Geometry check sheet. Reference: the model listing, model coordinates, mm. Face numbers are marked on the shaded views. A direction names the side the tool comes from. Round coordinates to 2 decimals unless told otherwise and drop trailing zeros. Loops run counter-clockwise (first coordinate to the right, second up) from the corner with the lowest first, then second, coordinate; pieces in that order, holes last.
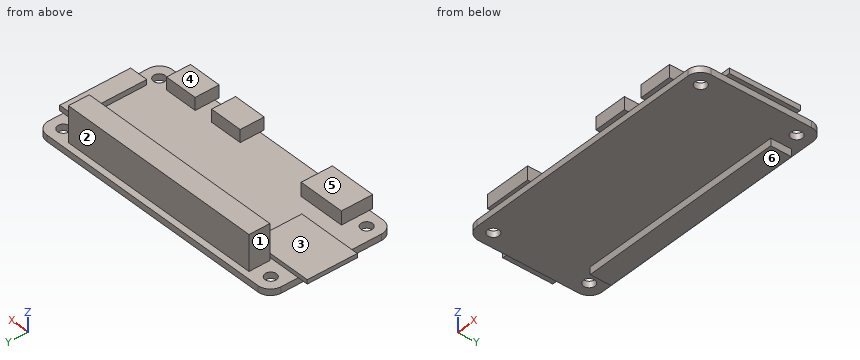
```python
from build123d import *

# Parameters (mm, degrees)
F0_W     = 8
F0_H     = 4.75
F0_W_2   = 11.25
F0_H_2   = 6.75
F0_W_3   = 3.5
F0_H_3   = 17
F0_W_4   = 13
F0_H_4   = 12
F0_R     = 1.375
F0_W_5   = 50.5
F0_H_5   = 5
F1_DEPTH = 1.5
F2_DEPTH = 3.25
F0_W_6   = 2.5
F3_DEPTH = 1
F0_H_6   = 0.75
F4_DEPTH = 3.25
F0_H_7   = 1
F5_DEPTH = 3
F0_W_7   = 1
F6_DEPTH = 1.25
F7_DEPTH = 8.5


with BuildPart() as f1:
    # F0 (on Top) → F1 (new body)
    with BuildSketch(Plane.XY):
        with Locations((21.5, -12.625)):
            Rectangle(F0_W, F0_H)
        with Locations((8.9, -12.625)):
            Rectangle(F0_W, F0_H)
        with Locations((-20.1, -11.625)):
            Rectangle(F0_W_2, F0_H_2)
        with Locations((30.75, 0)):
            Rectangle(F0_W_3, F0_H_3)
        with Locations((-26, 1.9)):
            Rectangle(F0_W_4, F0_H_4)
        with BuildLine():
            ThreePointArc((32.5, 12), (31.62132, 14.12132), (29.5, 15))
            Line((29.5, 15), (-29.5, 15))
            ThreePointArc((-29.5, 15), (-31.62132, 14.12132), (-32.5, 12))
            Line((-32.5, 12), (-32.5, 7.9))
            Line((-32.5, 7.9), (-19.5, 7.9))
            Line((-19.5, 7.9), (-19.5, -4.1))
            Line((-19.5, -4.1), (-32.5, -4.1))
            Line((-32.5, -4.1), (-32.5, -12))
            ThreePointArc((-32.5, -12), (-31.62132, -14.12132), (-29.5, -15))
            Line((-29.5, -15), (-25.725, -15))
            Line((-25.725, -15), (-25.725, -8.25))
            Line((-25.725, -8.25), (-14.475, -8.25))
            Line((-14.475, -8.25), (-14.475, -15))
            Line((-14.475, -15), (4.9, -15))
            Line((4.9, -15), (4.9, -10.25))
            Line((4.9, -10.25), (12.9, -10.25))
            Line((12.9, -10.25), (12.9, -15))
            Line((12.9, -15), (17.5, -15))
            Line((17.5, -15), (17.5, -10.25))
            Line((17.5, -10.25), (25.5, -10.25))
            Line((25.5, -10.25), (25.5, -15))
            Line((25.5, -15), (29.5, -15))
            ThreePointArc((29.5, -15), (31.62132, -14.12132), (32.5, -12))
            Line((32.5, -12), (32.5, -8.5))
            Line((32.5, -8.5), (29, -8.5))
            Line((29, -8.5), (29, 8.5))
            Line((29, 8.5), (32.5, 8.5))
            Line((32.5, 8.5), (32.5, 12))
        make_face()
        with Locations((-29, -11.5)):
            Circle(F0_R, mode=Mode.SUBTRACT)
        with Locations((29, -11.5)):
            Circle(F0_R, mode=Mode.SUBTRACT)
        with Locations((-29, 11.5)):
            Circle(F0_R, mode=Mode.SUBTRACT)
        with Locations((0, 11)):
            Rectangle(F0_W_5, F0_H_5, mode=Mode.SUBTRACT)
        with Locations((29, 11.5)):
            Circle(F0_R, mode=Mode.SUBTRACT)
        with Locations((0, 11)):
            Rectangle(F0_W_5, F0_H_5)
    extrude(amount=-F1_DEPTH)

    # F0 (on Top) → F2 (join)
    with BuildSketch(Plane.XY):
        with Locations((0, 11)):
            Rectangle(F0_W_5, F0_H_5)
    extrude(amount=-F2_DEPTH)

    # F0 (on Top) → F3 (join)
    with BuildSketch(Plane.XY):
        with Locations((-33.75, 1.9)):
            Rectangle(F0_W_6, F0_H_4)
        with Locations((-26, 1.9)):
            Rectangle(F0_W_4, F0_H_4)
    extrude(amount=F3_DEPTH)

    # F0 (on Top) → F4 (join)
    with BuildSketch(Plane.XY):
        with Locations((-20.1, -11.625)):
            Rectangle(F0_W_2, F0_H_2)
        with Locations((-20.1, -15.375)):
            Rectangle(F0_W_2, F0_H_6)
    extrude(amount=F4_DEPTH)

    # F0 (on Top) → F5 (join)
    with BuildSketch(Plane.XY):
        with Locations((8.9, -12.625)):
            Rectangle(F0_W, F0_H)
        with Locations((21.5, -12.625)):
            Rectangle(F0_W, F0_H)
        with Locations((21.5, -15.5)):
            Rectangle(F0_W, F0_H_7)
        with Locations((8.9, -15.5)):
            Rectangle(F0_W, F0_H_7)
    extrude(amount=F5_DEPTH)

    # F0 (on Top) → F6 (join)
    with BuildSketch(Plane.XY):
        with Locations((30.75, 0)):
            Rectangle(F0_W_3, F0_H_3)
        with Locations((33, 0)):
            Rectangle(F0_W_7, F0_H_3)
    extrude(amount=F6_DEPTH)

    # F0 (on Top) → F7 (join)
    with BuildSketch(Plane.XY):
        with Locations((0, 11)):
            Rectangle(F0_W_5, F0_H_5)
    extrude(amount=F7_DEPTH)


solid = f1.part
```
1) Sectioned sample at B-B, the plane y = 7. Record the cut outline in (x, z), then the cut area to 3 significant figures.
Report:
outline: (-35, 0) - (-32.5, 0) - (-32.5, -1.5) - (32.5, -1.5) - (32.5, 0) - (33.5, 0) - (33.5, 1.25) - (29, 1.25) - (29, 0) - (-19.5, 0) - (-19.5, 1) - (-35, 1) - close
area: 119 mm2
2) Mould release check, pull along Y, two halves, no side actions. Record for the marked faces 1, 2 and 3: +Y half, -Y half, draft (parallel to the pull), parting line (faces both ways), or undercut.
Report:
face 1: draft
face 2: +Y half
face 3: undercut
3) Sectioned sample at D-D, the plane z = 4.25. Record the cut outline in (x, y), then the cut area to 4 significant figures.
Report:
outline: (-25.25, 8.5) - (25.25, 8.5) - (25.25, 13.5) - (-25.25, 13.5) - close
area: 252.5 mm2
4) Gauge pin test, flat ends, axial feed: pin 1 (4 mm diameter, centred on x = 6.5, y = -8.5, fed in from +Z); pin 2 (1.5 mm diameter, centred on x = -10.5, z = 6.5, fed in from -Y); pin 3 (1.1 mm diameter, centred on x = -28.5, z = 0.5, fed in from -Y); pin 4 (2 mm diameter, centred on x = -29, y = -11.5, fed in from -Z). Record the tip position at first contact, or that the pin passes through.
Report:
pin 1: stops at z = 3
pin 2: stops at y = 8.5
pin 3: stops at y = -15
pin 4: passes through
5) Sectioned sample at A-A, the plane x = -11. Record the cut outline in (y, z).
Report:
outline: (-15, -1.5) - (8.5, -1.5) - (8.5, -3.25) - (13.5, -3.25) - (13.5, -1.5) - (15, -1.5) - (15, 0) - (13.5, 0) - (13.5, 8.5) - (8.5, 8.5) - (8.5, 0) - (-15, 0) - close
6) Sectioned sample at C-C, the plane x = 6.5. Record the cut outline in (y, z), then the cut area to 4 significant figures.
Report:
outline: (-16, 0) - (-15, 0) - (-15, -1.5) - (8.5, -1.5) - (8.5, -3.25) - (13.5, -3.25) - (13.5, -1.5) - (15, -1.5) - (15, 0) - (13.5, 0) - (13.5, 8.5) - (8.5, 8.5) - (8.5, 0) - (-10.25, 0) - (-10.25, 3) - (-16, 3) - close
area: 113.5 mm2
7) Access from +Z, -Z, +X, -X, +Y, -Y to the whole of each face (thin tool, end or side, straight path). Record for the marked faces 4, 5 and 6.
Report:
face 4: +Z, +X, -Y
face 5: +Z, +X, -X, -Y
face 6: -Z, +X, -X, +Y, -Y
8) Scan lines: line 1 along Y through (x, z) = (29, -1.05) (3 decimals); line 2 along X through (y, z) = (12.5, -0.75); line 3 along Z through (x, y) = (-12, -13). Record each from-to range of solid material in increasing order.
Report:
line 1: y = -15 to -12.875, -10.125 to 10.125, 12.875 to 15
line 2: x = -32.46 to -29.94, -28.06 to 28.06, 29.94 to 32.46
line 3: z = -1.5 to 0
